The model under review builds one solid part; all positions refer to its coordinate system, in mm. Coordinates: 2 decimals unless noted, no trailing zeros. Loops run counter-clockwise (first coordinate to the right, second up) from the corner with the lowest first, then second, coordinate; pieces in that order, holes last. Notation, with made-up numbers: M 28.5,19.25 L 85.5,19.25 A18 cw 85.5,51.25 Z; hole C 31,51.25 d7. An arc over 180 degrees is marked long. Return JSON: item names as keys, results as strings.
```python
from build123d import *

# Parameters (mm, degrees)
BOSS_EXTRUDE1_DEPTH = 4.5593
CAVITY1_START       = -112.395
CAVITY1_OUTLINE_W   = 4.5593
CAVITY1_OUTLINE_H   = 4.5593
CAVITY1_OUTLINE_W_2 = 31.27375
CAVITY1_DEPTH       = 4.5593
CAVITY1_START_2     = -49.8475
CAVITY1_2_OUTLINE_W = 4.5593
CAVITY1_2_OUTLINE_H = 4.5593
CAVITY1_2_DEPTH     = 31.27375
CAVITY1_START_3     = 12.7
CAVITY1_3_OUTLINE_W = 4.5593
CAVITY1_3_OUTLINE_H = 4.5593
CAVITY1_3_DEPTH     = 31.27375
CAVITY1_START_4     = 75.2475
CAVITY1_4_OUTLINE_W = 4.5593
CAVITY1_4_OUTLINE_H = 4.5593
CAVITY1_4_DEPTH     = 31.27375
CAVITY1_START_5     = -107.8357
CAVITY1_5_OUTLINE_W = 4.5593
CAVITY1_5_OUTLINE_H = 4.5593
CAVITY1_5_DEPTH     = 26.71445


# Read off the part's stored shape, not the designer's step: Cavity1
with BuildPart() as part:
    # Sketch1 → Boss-Extrude1 (new body)
    with BuildSketch(Plane.XY):
        Polygon((-112.395, -17.145), (-137.795, -17.145), (-137.795, -112.395), (112.395, -112.395), (112.395, 112.395), (112.395, 137.795), (17.145, 137.795), (17.145, 112.395), (-110.871, 112.395), (-110.871, 113.919), (-113.919, 113.919), (-113.919, 110.871), (-112.395, 110.871), align=None)
    extrude(amount=BOSS_EXTRUDE1_DEPTH)

    # Cavity1 outline → Cavity1 (cut)
    with BuildSketch(Plane(origin=(0, 0, 0), x_dir=(1, 0, 0), z_dir=(0, 1, 0)).offset(CAVITY1_START)):
        with Locations((110.11535, -2.27965)):
            Rectangle(CAVITY1_OUTLINE_W, CAVITY1_OUTLINE_H)
        with Locations((65.484375, -2.27965)):
            Rectangle(CAVITY1_OUTLINE_W_2, CAVITY1_OUTLINE_H)
        with Locations((2.936875, -2.27965)):
            Rectangle(CAVITY1_OUTLINE_W_2, CAVITY1_OUTLINE_H)
        with Locations((-59.610625, -2.27965)):
            Rectangle(CAVITY1_OUTLINE_W_2, CAVITY1_OUTLINE_H)
        with Locations((-122.158125, -2.27965)):
            Rectangle(CAVITY1_OUTLINE_W_2, CAVITY1_OUTLINE_H)
    extrude(amount=CAVITY1_DEPTH, mode=Mode.SUBTRACT)

    # Cavity1 2 outline → Cavity1 2 (cut)
    with BuildSketch(Plane(origin=(0, 0, 0), x_dir=(1, 0, 0), z_dir=(0, 1, 0)).offset(CAVITY1_START_2)):
        with Locations((110.11535, -2.27965)):
            Rectangle(CAVITY1_2_OUTLINE_W, CAVITY1_2_OUTLINE_H)
    extrude(amount=CAVITY1_2_DEPTH, mode=Mode.SUBTRACT)

    # Cavity1 3 outline → Cavity1 3 (cut)
    with BuildSketch(Plane(origin=(0, 0, 0), x_dir=(1, 0, 0), z_dir=(0, 1, 0)).offset(CAVITY1_START_3)):
        with Locations((110.11535, -2.27965)):
            Rectangle(CAVITY1_3_OUTLINE_W, CAVITY1_3_OUTLINE_H)
    extrude(amount=CAVITY1_3_DEPTH, mode=Mode.SUBTRACT)

    # Cavity1 4 outline → Cavity1 4 (cut)
    with BuildSketch(Plane(origin=(0, 0, 0), x_dir=(1, 0, 0), z_dir=(0, 1, 0)).offset(CAVITY1_START_4)):
        with Locations((110.11535, -2.27965)):
            Rectangle(CAVITY1_4_OUTLINE_W, CAVITY1_4_OUTLINE_H)
    extrude(amount=CAVITY1_4_DEPTH, mode=Mode.SUBTRACT)

    # Cavity1 5 outline → Cavity1 5 (cut)
    with BuildSketch(Plane(origin=(0, 0, 0), x_dir=(1, 0, 0), z_dir=(0, 1, 0)).offset(CAVITY1_START_5)):
        with Locations((110.11535, -2.27965)):
            Rectangle(CAVITY1_5_OUTLINE_W, CAVITY1_5_OUTLINE_H)
    extrude(amount=CAVITY1_5_DEPTH, mode=Mode.SUBTRACT)


solid = part.part
```
1. Add section B-B on x = -87. Give the boundary of the cut face in (y, z) (3 decimals).
Check values:
{"outline": "M -112.395,0 L 112.395,0 L 112.395,4.559 L -112.395,4.559 Z"}
2. Insertion check: pin 1 Ø1 at (x, z) = (74, 0.5) entering from -Y; pin 2 Ø1.4 at (y, z) = (-109, 2) entering from -X. Each pin has a flat end and moves straight along its axis. Give the tip position at first contact, or say it passes through.
Check values:
{"pin 1": "y = -107.84", "pin 2": "x = -106.52"}
3. Add section A-A on y = -89. Give the boundary of the cut face in (x, z) (3 decimals).
Check values:
{"outline": "M -137.795,0 L 107.836,0 L 107.836,4.559 L -137.795,4.559 Z"}
4. To check wall thickness, follow line 1 (Y direction, x = -24, z = 0.6) (3 decimals); line 2 (Y direction, x = -7, z = 2) (3 decimals). State the ranges of each line that lie inside material, in increasing order.
Check values:
{"line 1": "-112.395 to 112.395", "line 2": "-107.836 to 112.395"}
